from build123d import *

# Parameters (mm, degrees)
F0_W      = 23
F0_H      = 67
F1_DEPTH  = 11.2
F2_W      = 19
F2_H      = 63
F3_DEPTH  = 9.2
F4_W      = 12.1
F4_H      = 13.5
F5_DEPTH  = 12
F7_DEPTH  = 2
F9_DEPTH  = 1
F11_DEPTH = 1
F12_W     = 63
F12_H     = 1.9999997959
F13_DEPTH = 21
F14_DEPTH = 2
F15_W     = 7.9889474437
F15_H     = 3.3084521592
F16_DEPTH = 1


with BuildPart() as f1:
    # F0 (on Top) → F1 (new body)
    with BuildSketch(Plane.XY):
        with Locations((5.9262745458, 0)):
            Rectangle(F0_W, F0_H)
    extrude(amount=F1_DEPTH)

    # F2 (on face) → F3 (cut)
    with BuildSketch(Plane.XY.offset(11.2)):
        with Locations((5.9262745458, 0)):
            Rectangle(F2_W, F2_H)
    extrude(amount=-F3_DEPTH, mode=Mode.SUBTRACT)

    # F4 (on face) → F5 (cut)
    with BuildSketch(Plane.XZ.offset(33.5)):
        with Locations((5.9262745458, 11.2)):
            Rectangle(F4_W, F4_H)
    extrude(amount=-F5_DEPTH, mode=Mode.SUBTRACT)

    # F6 (on face) → F7 (cut)
    with BuildSketch(Plane(origin=(0, 33.5, 0), x_dir=(-1, 0, 0), z_dir=(0, 1, 0))):
        with BuildLine():
            ThreePointArc((-5.9262745458, 9.6), (-8.7547016705, 8.4284271247), (-9.9262745458, 5.6))
            Line((-9.9262745458, 5.6), (-5.9262745458, 5.6))
            Line((-5.9262745458, 5.6), (-5.9262745458, 9.6))
        make_face()
        with BuildLine():
            Line((-5.9262745458, 5.6), (-9.9262745458, 5.6))
            ThreePointArc((-9.9262745458, 5.6), (-8.7547016705, 2.7715728753), (-5.9262745458, 1.6))
            Line((-5.9262745458, 1.6), (-5.9262745458, 5.6))
        make_face()
        with BuildLine():
            Line((-5.9262745458, 9.6), (-5.9262745458, 5.6))
            Line((-5.9262745458, 5.6), (-1.9262745458, 5.6))
            ThreePointArc((-1.9262745458, 5.6), (-3.097847421, 8.4284271247), (-5.9262745458, 9.6))
        make_face()
        with BuildLine():
            Line((-1.9262745458, 5.6), (-5.9262745458, 5.6))
            Line((-5.9262745458, 5.6), (-5.9262745458, 1.6))
            ThreePointArc((-5.9262745458, 1.6), (-3.097847421, 2.7715728753), (-1.9262745458, 5.6))
        make_face()
    extrude(amount=-F7_DEPTH, mode=Mode.SUBTRACT)

    # F8 (on face) → F9 (cut)
    with BuildSketch(Plane.XY.offset(2)):
        Polygon((4.1827149684, 31.5), (1.9262745458, 31.5), (1.9262745458, 25.1600015908), (9.9262745458, 25.1600015908), (9.9262745458, 31.5), (7.6698341232, 31.5), align=None)
    extrude(amount=-F9_DEPTH, mode=Mode.SUBTRACT)

    # F10 (on face) → F11 (join)
    with BuildSketch(Plane.XY.offset(2)):
        Polygon((1.9262745458, 31.5), (-3.5737254542, 31.5), (-3.5737254542, -31.5), (15.4262745458, -31.5), (15.4262745458, 31.5), (9.9262745458, 31.5), (9.9262745458, 25.1600015908), (1.9262745458, 25.1600015908), align=None)
    extrude(amount=F11_DEPTH)

    # F12 (on face) → F13 (join)
    with BuildSketch(Plane.YZ.offset(-3.5737254542)):
        with Locations((0, 10.2000001021)):
            Rectangle(F12_W, F12_H)
    extrude(amount=F13_DEPTH)

    # F14 (add): a face of the model
    f14_faces = [f1.faces().sort_by_distance(p)[0] for p in [
        (5.9262745458, -31.5, 10.2000001021),
    ]]
    extrude(f14_faces, amount=F14_DEPTH)

    # F15 (on face) → F16 (cut)
    with BuildSketch(Plane(origin=(0, 0, 9.2000002041), x_dir=(1, 0, 0), z_dir=(0, 0, -1))):
        with Locations((5.9536970221, -29.8457739204)):
            Rectangle(F15_W, F15_H)
    extrude(amount=-F16_DEPTH, mode=Mode.SUBTRACT)


solid = f1.part
Work out the finished part from the listing and answer in its coordinate system (mm). A direction names the side the tool comes from. Coordinates: 2 decimals unless noted, no trailing zeros. Loops run counter-clockwise (first coordinate to the right, second up) from the corner with the lowest first, then second, coordinate; pieces in that order, holes last. Notation, with made-up numbers: M 84.25,-18.75 L 106.25,-18.75 A13 ccw 106.25,-3.75 Z; hole C 48,1 d10. An arc over 180 degrees is marked long. Answer in a Markdown table with one row per item. Add a question column.
1. Find section D-D, the plane z = 6.75. Write down the section's boundary in (x, y).
2. The mould has two halves that part along X. Classify faces 4 (the flat face through (-5.574, 0, 6)), 5 (the flat face through (6, -33.5, 4)), 6 (the flat face through (6, 28, 1)): pulls with the +X half, pulls with the -X half, needs draft (parallel to the pull), parting line crosses it, or undercut.
3. Find section A-A, the plane x = 13.25. Write down the section's boundary in (y, z), then the cut area to 3 significant figures.
4. Consider L1, parallel to Z at x = 14.5, y = 21; L2, parallel to X at y = 8, z = 9; L3, parallel to Y at x = 12, z = 4. Determine where each line is inside the solid, lowest interval first.
5. Find section C-C, the plane x = 3.75. Write down the section's boundary in (y, z), then the cut area to 3 significant figures.
6. A tool of negligible diameter and unlimited length cuts with its end or side. For faces 1 (the flat face through (6, 0, 11.2)), 2 (the flat face through (6, 31.5, 10)), 3 (the flat face through (-0.124, -33, 7)), from which of +Z, -Z, +X, -X, +Y, -Y can it reach the whole face along a straight path? Write none if from no direction.
7. A flat-ended cylindrical pin translates along its axis: P1, Ø5, axis at x = 6, z = 4.5, coming from the +Y side. Find the tip coordinate at first contact, or state that the pin passes through.
8. Find section B-B, the plane y = -14. Write down the section's boundary in (x, z).
Reported:
| question | item | result |
|---|---|---|
| 1 | outline | M -5.57,-33.5 L -0.12,-33.5 L -0.12,-31.5 L -3.57,-31.5 L -3.57,31.5 L 2.1,31.5 L 2.1,33.5 L -5.57,33.5 Z; M 9.76,31.5 L 15.43,31.5 L 15.43,-31.5 L 11.98,-31.5 L 11.98,-33.5 L 17.43,-33.5 L 17.43,33.5 L 9.76,33.5 Z |
| 2 | face 4 | pulls with the -X half |
| 2 | face 5 | needs draft |
| 2 | face 6 | undercut |
| 3 | outline | M -33.5,0 L 33.5,0 L 33.5,11.2 L -33.5,11.2 Z; hole M -31.5,3 L 31.5,3 L 31.5,9.2 L -31.5,9.2 Z |
| 3 | area | 360 mm^2 |
| 4 | L1 | z = 0 to 3, 9.2 to 11.2 |
| 4 | L2 | x = -5.57 to -3.57, 15.43 to 17.43 |
| 4 | L3 | y = -33.5 to -31.5, 31.5 to 33.5 |
| 5 | outline | M -33.5,0 L 33.5,0 L 33.5,2.24 L 31.5,2.24 L 31.5,1 L 25.16,1 L 25.16,3 L -31.5,3 L -31.5,4.45 L -33.5,4.45 Z; M -33.5,9.2 L 28.19,9.2 L 28.19,10.2 L 31.5,10.2 L 31.5,8.96 L 33.5,8.96 L 33.5,11.2 L -33.5,11.2 Z |
| 5 | area | 321 mm^2 |
| 6 | face 1 | +Z, +X, -X, +Y, -Y |
| 6 | face 2 | none |
| 6 | face 3 | -Y |
| 7 | P1 | stops at y = 25.16 |
| 8 | outline | M -5.57,0 L 17.43,0 L 17.43,11.2 L -5.57,11.2 Z; hole M -3.57,3 L 15.43,3 L 15.43,9.2 L -3.57,9.2 Z |
